Input: part model. Units: mm. Frame: model coordinates. Face numbers are marked on the shaded views. A direction names the side the tool comes from. Round coordinates to 2 decimals unless told otherwise and drop trailing zeros. Loops run counter-clockwise (first coordinate to the right, second up) from the corner with the lowest first, then second, coordinate; pieces in that order, holes last. Notation, with made-up numbers: (-29.75, 16) - (1.25, 16) arc R29 cw to (1.25, 47) - close; hole circle Ø10 at (-18, 82). An arc over 180 degrees is marked (long way). Write each question's results on one line, items separated by ' | '.
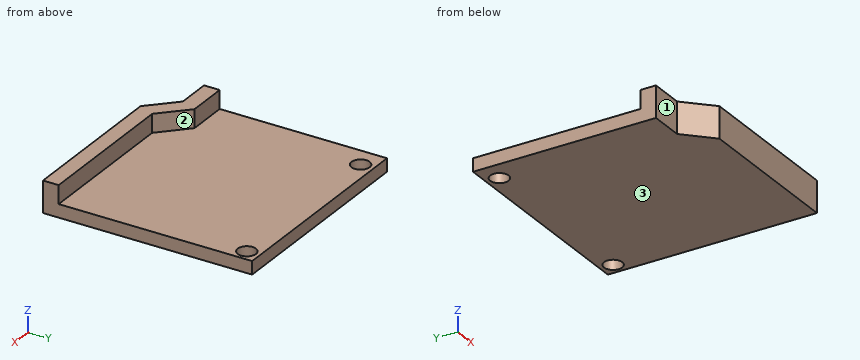
Autodesk Inventor part; units mm, degrees
ref_plane "YZ Plane" through (0, 0, 0) normal (1, 0, 0) x (0, 1, 0)
ref_plane "XZ Plane" through (0, 0, 0) normal (0, 1, 0) x (-1, 0, 0)
ref_plane "XY Plane" through (0, 0, 0) normal (0, 0, 1) x (1, 0, 0)
sketch "Sketch4" plane through (0, 0, 0) normal (0, 0, 1) x (1, 0, 0)
  line L0 (0, 0) -> (30, 0)
  line L1 (0, 0) -> (-5, 5)
  line L2 (-5, 5) -> (-11.5, 5)
  line L3 (30, 0) -> (30, 40)
  line L4 (30, 40) -> (-11.5, 40)
  line L5 (-11.5, 40) -> (-11.5, 5)
  dimension "d16" = 30
  dimension "d17" = 5
  dimension "d18" = 135
  dimension "d19" = 6.5
  dimension "d20" = 40
extrude "Extrusion4" add sketch "Sketch4" along normal blind 2.5
sketch "Sketch5" plane through (0, 0, 2.5) normal (0, 0, 1) x (1, 0, 0)
  line L0 (0, 0) -> (30, 0)
  line L1 (30, 0) -> (30, 40)
  line L2 (-11.5, 40) -> (-11.5, 5)
  line L3 (-11.5, 5) -> (-5, 5)
  line L4 (-5, 5) -> (0, 0)
  line L5 (-11.5, 8) -> (-3.7574, 8)
  line L6 (-3.7574, 8) -> (1.2426, 3)
  line L7 (1.2426, 3) -> (30, 3)
  dimension "d23" = 3
  dimension "d24" = 3
  dimension "d25" = 3
extrude "Extrusion5" add sketch "Sketch5" along normal blind 3.5
sketch "Sketch6" plane through (0, 0, 2.5) normal (0, 0, 1) x (1, 0, 0)
  line L0 (-11.5, 8) -> (-3.7574, 8)
  line L1 (1.2426, 3) -> (30, 3)
  line L2 (30, 3) -> (30, 40)
  line L3 (-11.5, 40) -> (-11.5, 8)
  circle A0 centre (-7.4, 37.5) radius 1.75
  circle A1 centre (27.6, 37.5) radius 1.75
  point P0 (0, 0)
  dimension "d28" = 29.5
  dimension "d29" = 4.1
  dimension "d30" = 3.5
  dimension "d31" = 3.5
  dimension "d32" = 2.4
  dimension "d33" = 34.5
  dimension "d36" = 6
  dimension "d37" = 6
extrude "Extrusion6" cut sketch "Sketch6" against normal up to next
properties part number "XCarriageFanMount"
1. Section query D-D, the plane z = 1.8. Output: boundary loops of the cut face in (x, y), plus the area to 3 significant figures.
Answer:
outline: (-11.5, 5) - (-5, 5) - (0, 0) - (30, 0) - (30, 40) - (-11.5, 40) - close; hole circle Ø3.5 at (-7.4, 37.5); hole circle Ø3.5 at (27.6, 37.5) | area: 1,600 mm^2
2. Section query C-C, the plane z = 4.75. Output: boundary loops of the cut face in (x, y).
Answer:
outline: (-11.5, 5) - (-5, 5) - (0, 0) - (30, 0) - (30, 3) - (1.24, 3) - (-3.76, 8) - (-11.5, 8) - close
3. Set-up query: the marked faces 1, 2 and 3. Return all of +Z, -Z, +X, -X, +Y, -Y with unobstructed straight access to the full face (end or side cutting, diameter ignored); none if empty.
Answer:
face 1: +Z, -Z, -X, -Y | face 2: +Z, +X, +Y | face 3: -Z, +X, -X, +Y, -Y
4. Contact query for flat-ended pins moving along their axis: pin 1 (3 mm diameter, centred on x = -8, z = 1.5, fed in from -Y); pin 2 (10 mm diameter, centred on x = 5.5, y = 10, fed in from +Z); pin 3 (3 mm diameter, centred on x = -6.5, y = 12.5, fed in from -Z); pin 4 (1.8 mm diameter, centred on x = -7.5, z = 4, fed in from +Y). Output: stop coordinate, or through.
Answer:
pin 1: y = 5 | pin 2: z = 2.5 | pin 3: z = 0 | pin 4: y = 8
5. Line query: line 1 (Y direction, x = 27.6, z = 1.4); line 2 (Y direction, x = -7.4, z = 0.6); line 3 (Z direction, x = -8, y = 20). Output: solid intervals per line, ascending. Write a range as [from, to].
Answer:
line 1: [0, 35.75], [39.25, 40] | line 2: [5, 35.75], [39.25, 40] | line 3: [0, 2.5]
6. Section query A-A, the plane y = 37.5. Output: boundary loops of the cut face in (x, z).
Answer:
outline: (-11.5, 0) - (-9.15, 0) - (-9.15, 2.5) - (-11.5, 2.5) - close; (-5.65, 0) - (25.85, 0) - (25.85, 2.5) - (-5.65, 2.5) - close; (29.35, 0) - (30, 0) - (30, 2.5) - (29.35, 2.5) - close
7. Section query B-B, the plane x = -7.4. Output: boundary loops of the cut face in (y, z).
Answer:
outline: (5, 0) - (35.75, 0) - (35.75, 2.5) - (8, 2.5) - (8, 6) - (5, 6) - close; (39.25, 0) - (40, 0) - (40, 2.5) - (39.25, 2.5) - close
